Geometry: final body of the model. Coordinates: model frame, mm. A direction names the side the tool comes from. Give positions to 0.01 mm unless a question says otherwise; leave off trailing zeros. Order: outer loops, then holes, each group sorted by start corner. A loop starts at its lowest first (then second) coordinate and runs counter-clockwise, first axis right, second up. Notation, with made-up numbers: (87, 22.25) - (93, 22.25) arc R30 ccw to (93, 49.25) - close; hole circle Ø1 at (64.5, 13). An arc over 180 degrees is marked (long way). One line per item, written item: value.
```python
from build123d import *

# Parameters (mm, degrees)
F0_W     = 37.5
F0_H     = 10
F0_R     = 5
F1_DEPTH = 63
F2_R     = 5
F3_DEPTH = 10
F5_DEPTH = 53
F7_DEPTH = 63
F9_DEPTH = 25


with BuildPart() as f1:
    # F0 (on Front) → F1 (new body)
    with BuildSketch(Plane.XZ):
        Polygon((-5, 0), (0, 0), (5, 0), (5, 10), (-5, 10), align=None)
        with Locations((-23.75, 5)):
            Rectangle(F0_W, F0_H)
        with Locations((23.75, 5)):
            Rectangle(F0_W, F0_H)
        with BuildLine():
            Line((-42.5, 10), (-5, 10))
            Line((-5, 10), (-5, 40.72949))
            ThreePointArc((-5, 40.72949), (-14.455244, 47.63613), (-17.439102, 58.95867))
            Line((-17.439102, 58.95867), (-42.5, 10))
        make_face()
        with BuildLine():
            Line((5, 40.72949), (5, 10))
            Line((5, 10), (42.5, 10))
            Line((42.5, 10), (17.439102, 58.95867))
            ThreePointArc((17.439102, 58.95867), (17.484769, 58.22997), (17.5, 57.5))
            ThreePointArc((17.5, 57.5), (14.031215, 47.04175), (5, 40.72949))
        make_face()
        with BuildLine():
            ThreePointArc((-17.439102, 58.95867), (-14.455244, 47.63613), (-5, 40.72949))
            ThreePointArc((-5, 40.72949), (0, 40), (5, 40.72949))
            ThreePointArc((5, 40.72949), (14.031215, 47.04175), (17.5, 57.5))
            ThreePointArc((17.5, 57.5), (17.484769, 58.22997), (17.439102, 58.95867))
            ThreePointArc((17.439102, 58.95867), (0, 75), (-17.439102, 58.95867))
        make_face()
        with Locations((0, 57.5)):
            Circle(F0_R, mode=Mode.SUBTRACT)
    extrude(amount=F1_DEPTH)

    # F2 (on Top) → F3 (cut)
    with BuildSketch(Plane.XY):
        with Locations((-22.5, -25)):
            Circle(F2_R)
        with Locations((22.5, -25)):
            Circle(F2_R)
    extrude(amount=F3_DEPTH, mode=Mode.SUBTRACT)

    # F4 (on face) → F5 (cut)
    with BuildSketch(Plane(origin=(0, 0, 0), x_dir=(-1, 0, 0), z_dir=(0, 1, 0))):
        with BuildLine():
            Line((-17.439102, 58.95867), (-42.5, 10))
            Line((-42.5, 10), (-5, 10))
            Line((-5, 10), (-5, 40.72949))
            ThreePointArc((-5, 40.72949), (-14.579622, 47.551258), (-17.439102, 58.95867))
        make_face()
        with BuildLine():
            Line((42.5, 10), (17.439102, 58.95867))
            ThreePointArc((17.439102, 58.95867), (14.579622, 47.551258), (5, 40.72949))
            Line((5, 40.72949), (5, 10))
            Line((5, 10), (42.5, 10))
        make_face()
    extrude(amount=-F5_DEPTH, mode=Mode.SUBTRACT)

    # F6 (on face) → F7 (join)
    with BuildSketch(Plane.XZ.offset(63)):
        with BuildLine():
            Line((-5, 40.72949), (-5, 10))
            Line((-5, 10), (5, 10))
            Line((5, 10), (5, 40.72949))
            ThreePointArc((5, 40.72949), (0, 40), (-5, 40.72949))
        make_face()
    extrude(amount=-F7_DEPTH)

    # F8 (on face) → F9 (cut, symmetric)
    with BuildSketch(Plane.YZ.offset(5)):
        Polygon((-15, 40.72949), (0, 10), (0, 75), (-15, 75), align=None)
    extrude(amount=F9_DEPTH, both=True, mode=Mode.SUBTRACT)


solid = f1.part
```
1) Section D-D, the plane z = 57.5. Return loops of the section in (x, y), then the cut area to 3 significant figures.
Answers below:
outline: (-18.19, -63) - (-5, -63) - (-5, -15) - (-17.53, -15) - (-17.53, -53) - (-18.19, -53) - close; (5, -63) - (18.19, -63) - (18.19, -53) - (17.53, -53) - (17.53, -15) - (5, -15) - close
area: 1,220 mm^2
2) First-contact query: pin 1 (9 mm diameter, centred on x = -22.5, y = -25, fed in from +Z); pin 2 (6 mm diameter, centred on y = -39, z = 61, fed in from -X); pin 3 (11 mm diameter, centred on x = 21, y = -26, fed in from +Z); pin 4 (9 mm diameter, centred on y = -28, z = 26.5, fed in from +X). Flat tips, straight axial feed; report the tip coordinate or a pass-through.
Answers below:
pin 1: through
pin 2: x = -17.52
pin 3: z = 65.62
pin 4: x = 5
3) Set-up query: faces 4 (the face through (5, -33, 25)), 5 (the face through (-28, -26, 10)), 6 (the face through (30.145, -57.93, 34.137)), 7 (the face through (4, -15, 54)), 8 (the face through (-42.5, -31, 5)). Return all of +Z, -Z, +X, -X, +Y, -Y with unobstructed straight access to the full face (end or side cutting, diameter ignored); none if empty.
Answers below:
face 4: +X, +Y
face 5: -X, +Y
face 6: +Z, +X, +Y, -Y
face 7: +Z, +X, -X, +Y
face 8: +Z, -Z, -X, +Y, -Y
4) Section A-A, the plane y = -25. Return loops of the section in (x, z).
Answers below:
outline: (-42.5, 0) - (-27.5, 0) - (-27.5, 10) - (-42.5, 10) - close; (-17.5, 0) - (17.5, 0) - (17.5, 10) - (5, 10) - (5, 40.73) arc R17 ccw to (17.44, 58.96) arc R17.5 ccw to (-17.44, 58.96) arc R17 ccw to (-5, 40.73) - (-5, 10) - (-17.5, 10) - close; (27.5, 0) - (42.5, 0) - (42.5, 10) - (27.5, 10) - close; hole circle Ø10 at (0, 57.5)
5) Section B-B, the plane x = 0. Return loops of the section in (y, z).
Answers below:
outline: (-63, 0) - (0, 0) - (0, 10) - (-15, 40.73) - (-15, 52.5) - (-63, 52.5) - close; (-63, 62.5) - (-15, 62.5) - (-15, 75) - (-63, 75) - close
6) Material intervals for line 1 along Z through (x, y) = (0.5, -29); line 2 along Y through (x, z) = (-22, 6); line 3 along X through (y, z) = (-37.5, 57.5), sorted ascending.
Answers below:
line 1: 0 to 52.53, 62.47 to 74.99
line 2: -63 to -29.97, -20.03 to 0
line 3: -17.53 to -5, 5 to 17.53
7) Mould query, pull axis Y, two halves, no side actions, for faces 1 (the face through (-29.794, -57.93, 34.822)), 2 (the face through (21.42, -29.88, 4.93)), 3 (the face through (-1, 0, 5)). Classes: released by +Y, released by -Y, zero draft, split by the parting line, or undercut.
Answers below:
face 1: zero draft
face 2: undercut
face 3: released by +Y
8) Section C-C, the plane y = -37. Return loops of the section in (x, z).
Answers below:
outline: (-42.5, 0) - (42.5, 0) - (42.5, 10) - (5, 10) - (5, 40.73) arc R17 ccw to (17.44, 58.96) arc R17.5 ccw to (-17.44, 58.96) arc R17 ccw to (-5, 40.73) - (-5, 10) - (-42.5, 10) - close; hole circle Ø10 at (0, 57.5)
